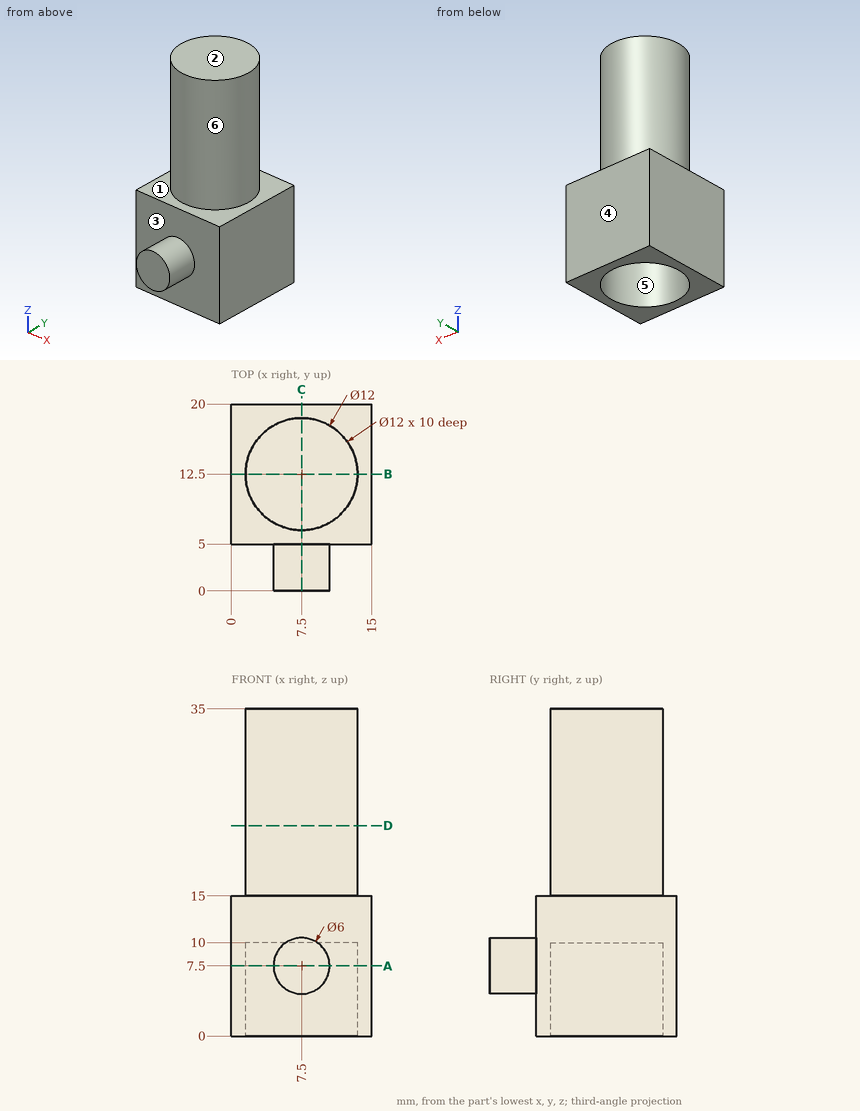
Verification items for this drawing (mm, ordinates from the low corner). A direction names the side the tool comes from. Coordinates: 2 decimals unless noted, no trailing zeros. Loops run counter-clockwise (first coordinate to the right, second up) from the corner with the lowest first, then second, coordinate; pieces in that order, holes last. Notation, with made-up numbers: (8.5, 9.5) - (49.5, 9.5) arc R35 ccw to (49.5, 47.5) - close; hole circle Ø5 at (55, 28.5). An arc over 180 degrees is marked (long way). Use one line per item in the form item = value. Start each with the question number.
Item 1: Section check D-D, the plane z = 22.5. Enter the section's corners in (x, y), and give its area (3 significant figures).
Item 2: Thickness scan on probe 1 along X at (y, z) = (12.5, 6.5); probe 2 along Y at (x, z) = (7.5, 7); probe 3 along Y at (x, z) = (7.5, 3). Record the ranges inside material, lowest first.
Item 3: Section check C-C, the plane x = 7.5. Enter the section's corners in (y, z), and give its area (3 significant figures).
Item 4: Section check B-B, the plane y = 12.5. Enter the section's corners in (x, z).
Item 5: Mould release check, pull along X, two halves, no side actions. Record for the marked faces 4, 5 and 6: +X half, -X half, draft (parallel to the pull), parting line (faces both ways), or undercut.
Item 6: Tool access check on the marked faces 1, 2 and 3. Record the directions out of +Z, -Z, +X, -X, +Y, -Y that give a thin tool (end or side, any length) a straight path to the whole face; none if there is none.
Item 7: Section check A-A, the plane z = 7.5. Enter the section's corners in (x, y).
Item 8: Gauge pin test, flat ends, axial feed: pin 1 (5 mm diameter, centred on y = 7.5, z = 20.5, fed in from -X); pin 2 (1.5 mm diameter, centred on x = 5, z = 14, fed in from -Y); pin 3 (3 mm diameter, centred on x = 6.5, y = 11.5, fed in from -Z). Record the tip position at first contact, or that the pin passes through.
Computed:
q1.outline = circle Ø12 at (7.5, 12.5)
q1.area = 113 mm2
q2.probe_1 = 0 to 1.5, 13.5 to 15
q2.probe_2 = 0 to 6.5, 18.5 to 20
q2.probe_3 = 5 to 6.5, 18.5 to 20
q3.outline = (0, 4.5) - (5, 4.5) - (5, 0) - (6.5, 0) - (6.5, 10) - (18.5, 10) - (18.5, 0) - (20, 0) - (20, 15) - (18.5, 15) - (18.5, 35) - (6.5, 35) - (6.5, 15) - (5, 15) - (5, 10.5) - (0, 10.5) - close
q3.area = 375 mm2
q4.outline = (0, 0) - (1.5, 0) - (1.5, 10) - (13.5, 10) - (13.5, 0) - (15, 0) - (15, 15) - (13.5, 15) - (13.5, 35) - (1.5, 35) - (1.5, 15) - (0, 15) - close
q5.face_4 = draft
q5.face_5 = undercut
q5.face_6 = parting line
q6.face_1 = +Z
q6.face_2 = +Z, +X, -X, +Y, -Y
q6.face_3 = -Y
q7.outline = (0, 5) - (4.5, 5) - (4.5, 0) - (10.5, 0) - (10.5, 5) - (15, 5) - (15, 20) - (0, 20) - close; hole circle Ø12 at (7.5, 12.5)
q8.pin_1 = 2.05
q8.pin_2 = 5
q8.pin_3 = 10
